CAD build for the part. Positions are in the model's coordinates, mm. A direction names the side the tool comes from. Coordinates: 2 decimals unless noted, no trailing zeros. Order: outer loops, then holes, each group sorted by start corner. A loop starts at its lowest first (then second) coordinate and runs counter-clockwise, first axis right, second up. Notation, with made-up numbers: (79.5, -6) - (128.5, -6) arc R34 ccw to (128.5, 30) - close; hole circle Ø7 at (-2, 34). An arc over 180 degrees is marked (long way). Write each question's results on one line, items separated by ' | '. Start each with the question number.
Q1. Wall check: probe 1 along Y at (x, z) = (20, 0.75); probe 2 along Y at (x, z) = (0, 1); probe 3 along Z at (x, y) = (-6.5, 1). Give the ranges that are in metal, low to high.
Q2. Pin check, flat tip, straight feed: P1, Ø6, axis at x = 8.5, z = 16, coming from the +Y side. Stop position of the tip, or through.
Q3. Band-saw the part on C-C, the plane z = 12. Write the cut outline in (x, y), then the cut area to 3 significant figures.
Q4. Pull direction X, two halves, no side cores. Call faces 3 (the cylindrical face through (-8, -5.4, 0.8)), 4 (the flat face through (25, -6.6, 0.5)), 5 (the flat face through (0, 1, 1.5)): released by +X, released by -X, zero draft, split by the parting line, or undercut.
Q5. Band-saw the part on A-A, the plane y = 0. Write the cut outline in (x, z), then the cut area to 3 significant figures.
Q6. Which spindle directions (+Z, -Z, +X, -X, +Y, -Y) get a long thin tool onto all of the face, cutting with end or side? Do faces 1 (the flat face through (0, -13.5, 16)), 2 (the flat face through (0, -15, 15)). Say none if no direction does.
Q7. Band-saw the part on D-D, the plane x = -20. Write the cut outline in (y, z).
Q8. Band-saw the part on B-B, the plane x = 0. Write the cut outline in (y, z) (3 decimals), then the cut area to 4 significant figures.
Autodesk Inventor part; units mm, degrees
ref_plane "YZ Plane" through (0, 0, 0) normal (1, 0, 0) x (0, 1, 0)
ref_plane "XZ Plane" through (0, 0, 0) normal (0, 1, 0) x (-1, 0, 0)
ref_plane "XY Plane" through (0, 0, 0) normal (0, 0, 1) x (1, 0, 0)
sketch "Sketch7" plane through (0, 0, 0) normal (0, 0, 1) x (1, 0, 0)
  line L0 (25, -15) -> (-25, -15)
  line L1 (-25, -15) -> (-25, 15)
  line L2 (-25, 15) -> (25, 15)
  line L3 (25, 15) -> (25, -15)
  line L4 (25, -15) -> (-25, 15) construction
  line L5 (-25, -15) -> (25, 15) construction
  point P0 (0, 0)
  dimension "d37" = 50
  dimension "d38" = 30
extrude "Extrusion4" add sketch "Sketch7" along normal blind 1.5
sketch "Sketch8" plane through (0, 0, 1.5) normal (0, 0, 1) x (1, 0, 0)
  line L0 (-25, -15) -> (25, -15)
  line L1 (-25, 15) -> (-25, -15)
  line L2 (25, -15) -> (-25, -15)
  line L3 (-25, -15) -> (-25, -13.5)
  line L4 (-25, -13.5) -> (25, -13.5)
  line L5 (25, -13.5) -> (25, -15)
  point P0 (0, 0)
  dimension "d41" = 1.5
extrude "Extrusion5" add sketch "Sketch8" along normal blind 28.5
sketch "Sketch14" plane through (0, 0, 0) normal (0, 0, -1) x (-1, 0, 0)
  circle A0 centre (0, 0) radius 8.5
  line L0 (-1.5, 8.3666) -> (-1.5, 10.3666)
  line L1 (-1.5, 8.3666) -> (0.5, 8.3666) construction
  line L2 (1.5, 8.3666) -> (1.5, 10.3666)
  arc A1 (1.5, 10.3666) -> (-1.5, 10.3666) centre (0, 10.3666) ccw
  line L3 (-6.4957, -5.4823) -> (-8.2277, -6.4823)
  arc A2 (-9.7277, -3.8843) -> (-8.2277, -6.4823) centre (-8.9777, -5.1833) ccw
  line L4 (-7.9957, -2.8843) -> (-9.7277, -3.8843)
  line L5 (7.9957, -2.8843) -> (9.7277, -3.8843)
  arc A3 (8.2277, -6.4823) -> (9.7277, -3.8843) centre (8.9777, -5.1833) ccw
  line L6 (6.4957, -5.4823) -> (8.2277, -6.4823)
  line L7 (-25, 15) -> (-25, -15)
  line L8 (25, -15) -> (25, 15)
  point P0 (-20, 0)
  point P1 (20, 0)
  dimension "d80" = 17
  dimension "d127" = 2
  dimension "d128" = 90
  dimension "d131" = 360
  dimension "d146" = 5
  dimension "d147" = 5
hole "Hole5" at (0, 10.3666, 0) at (-8.9777, -5.1833, 0) at (8.9777, -5.1833, 0) direction (0, 0, 1) diameter 2 end through all
hole "Hole6" at (-20, 0, 0) at (20, 0, 0) direction (0, 0, 1) diameter 3 end through all
sketch "Sketch17" plane through (0, -15, 17.5917) normal (0, -1, 0) x (-1, 0, 0)
  circle A0 centre (0, 0) radius 8.5
  line L0 (-1.5, 8.3666) -> (-1.5, 10.3666)
  line L1 (-1.5, 8.3666) -> (0.5, 8.3666) construction
  line L2 (1.5, 8.3666) -> (1.5, 10.3666)
  arc A1 (1.5, 10.3666) -> (-1.5, 10.3666) centre (0, 10.3666) ccw
  line L3 (-6.4957, -5.4823) -> (-8.2277, -6.4823)
  arc A2 (-9.7277, -3.8843) -> (-8.2277, -6.4823) centre (-8.9777, -5.1833) ccw
  line L4 (-7.9957, -2.8843) -> (-9.7277, -3.8843)
  line L5 (7.9957, -2.8843) -> (9.7277, -3.8843)
  arc A3 (8.2277, -6.4823) -> (9.7277, -3.8843) centre (8.9777, -5.1833) ccw
  line L6 (6.4957, -5.4823) -> (8.2277, -6.4823)
  line L7 (-25, 15) -> (-25, -15)
  line L8 (25, -15) -> (25, 15)
  point P0 (-20, 0)
  point P1 (20, 0)
  dimension "d155" = 17
  dimension "d154" = 2
  dimension "d169" = 90
  dimension "d151" = 360
  dimension "d153" = 5
  dimension "d152" = 5
hole "Hole10" at (0, -15, 7.225) at (-8.9777, -15, 22.775) at (8.9777, -15, 22.775) direction (0, 1, 0) diameter 2 end through all
hole "Hole11" at (-20, -15, 17.5917) at (20, -15, 17.5917) direction (0, 1, 0) diameter 3 end through all
properties part number "bracket_design2" material "Aluminum 6061"
Results below:
1) probe 1: y = -15 to -1.5, 1.5 to 15 | probe 2: y = -15 to 9.37, 11.37 to 15 | probe 3: z = 0 to 1.5
2) P1: stops at y = -13.5
3) outline: (-25, -15) - (25, -15) - (25, -13.5) - (-25, -13.5) - close | area: 75.0 mm²
4) face 3: undercut | face 4: released by +X | face 5: zero draft
5) outline: (-25, 0) - (-21.5, 0) - (-21.5, 1.5) - (-25, 1.5) - close; (-18.5, 0) - (18.5, 0) - (18.5, 1.5) - (-18.5, 1.5) - close; (21.5, 0) - (25, 0) - (25, 1.5) - (21.5, 1.5) - close | area: 66.0 mm²
6) face 1: +Z, +X, -X, +Y | face 2: +Z, -Z, +X, -X, -Y
7) outline: (-15, 0) - (-1.5, 0) - (-1.5, 1.5) - (-13.5, 1.5) - (-13.5, 16.09) - (-15, 16.09) - close; (-15, 19.09) - (-13.5, 19.09) - (-13.5, 30) - (-15, 30) - close; (1.5, 0) - (15, 0) - (15, 1.5) - (1.5, 1.5) - close
8) outline: (-15, 0) - (9.367, 0) - (9.367, 1.5) - (-13.5, 1.5) - (-13.5, 6.225) - (-15, 6.225) - close; (-15, 8.225) - (-13.5, 8.225) - (-13.5, 30) - (-15, 30) - close; (11.367, 0) - (15, 0) - (15, 1.5) - (11.367, 1.5) - close | area: 81.75 mm²
